```python
from build123d import *

# Parameters (mm, degrees)
SKETCH1_R           = 7.5
SKETCH1_R_2         = 4.5
BOSS_EXTRUDE1_DEPTH = 4
SKETCH3_W           = 1.525
SKETCH3_H           = 4
CUT_EXTRUDE1_DEPTH  = 1.075
CIRPATTERN1_COUNT   = 4
SKETCH6_R           = 0.75
CUT_EXTRUDE3_DEPTH  = 5
CIRPATTERN3_COUNT   = 4


with BuildPart() as part:
    # Sketch1 → Boss-Extrude1 (new body)
    with BuildSketch(Plane(origin=(0, 0, 0), x_dir=(1, 0, 0), z_dir=(0, 1, 0))):
        Circle(SKETCH1_R)
        Circle(SKETCH1_R_2, mode=Mode.SUBTRACT)
    extrude(amount=BOSS_EXTRUDE1_DEPTH)

    # Sketch3 → Cut-Extrude1 (cut, symmetric)
    with BuildSketch(Plane(origin=(0, 0, 0), x_dir=(0, 0, -1), z_dir=(1, 0, 0))):
        with Locations((-6.7375, 2)):
            Rectangle(SKETCH3_W, SKETCH3_H)
    cut_extrude1 = extrude(amount=CUT_EXTRUDE1_DEPTH, both=True, mode=Mode.SUBTRACT)

    # CirPattern1: Cut-Extrude1 ×4 about axis
    cirpattern1_axis = Axis((0, 0, 0), (0, 1, 0))
    for i in range(1, CIRPATTERN1_COUNT):
        add(cut_extrude1.rotate(cirpattern1_axis, i * 360 / CIRPATTERN1_COUNT), mode=Mode.SUBTRACT)

    # Sketch6 → Cut-Extrude3 (cut, through all)
    with BuildSketch(Plane.XZ):
        with Locations((4.242640687, 4.242640687)):
            Circle(SKETCH6_R)
    cut_extrude3 = extrude(amount=-CUT_EXTRUDE3_DEPTH, mode=Mode.SUBTRACT)

    # CirPattern3: Cut-Extrude3 ×4 about axis
    cirpattern3_axis = Axis((0, 0, 0), (0, 1, 0))
    for i in range(1, CIRPATTERN3_COUNT):
        add(cut_extrude3.rotate(cirpattern3_axis, i * 360 / CIRPATTERN3_COUNT), mode=Mode.SUBTRACT)


solid = part.part
```
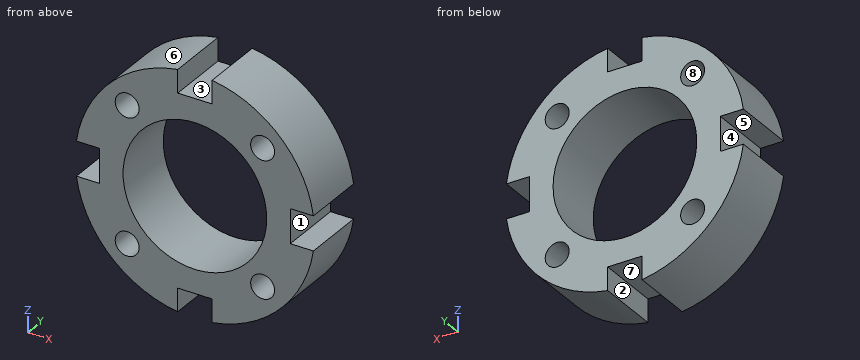
Part model, mm, in its own coordinate system. Face numbers are marked on the shaded views. A direction names the side the tool comes from. Round coordinates to 2 decimals unless told otherwise and drop trailing zeros. Loops run counter-clockwise (first coordinate to the right, second up) from the corner with the lowest first, then second, coordinate; pieces in that order, holes last. Notation, with made-up numbers: (-29.5, 63.5) -> (18.5, 63.5) arc R25 ccw to (18.5, 92.5) -> close; hole circle Ø5 at (76.25, 31.25). An arc over 180 degrees is marked (long way). Use one line per item in the form item = value. Start each with the question number.
Item 1: Two-plate mould, pull along X, no slides. Class the marked faces 5, 6, 7 and 8: released by +X, released by -X, zero draft, split by the parting line, or undercut.
Item 2: Band-saw the part on B-B (x = 0). List the corners of the cut face in (y, z) (3 decimals).
Item 3: Drop flat-ended pins along their axis: pin 1 Ø1.2 at (x, z) = (-4.24, -4.24) entering from -Y; pin 2 Ø1.7 at (y, z) = (2.5, 0.5) entering from +X; pin 3 Ø1.6 at (x, y) = (-6.5, 2.5) entering from +Z; pin 4 Ø0.6 at (x, y) = (0.5, 2) entering from -Z (3 decimals). Give the stop position or say it passes through.
Item 4: Drill centre lines: line 1 along X through (y, z) = (2.45, 4.75); line 2 along X through (y, z) = (0.85, -4). Where is each one in solid material? Low to high.
Item 5: Band-saw the part on C-C (y = 0.75). List the corners of the cut face in (x, z) (3 decimals).
Item 6: Band-saw the part on A-A (z = 0). List the corners of the cut face in (x, y) (3 decimals).
Item 7: Tool access for the marked faces 1, 2, 3 and 4: list every direction of +Z, -Z, +X, -X, +Y, -Y with a clear straight run to the whole face (end or side of a thin tool).
Data:
q1.face_5 = zero draft
q1.face_6 = released by -X
q1.face_7 = undercut
q1.face_8 = undercut
q2.outline = (0, -5.975) -> (4, -5.975) -> (4, -4.5) -> (0, -4.5) -> close; (0, 4.5) -> (4, 4.5) -> (4, 5.975) -> (0, 5.975) -> close
q3.pin_1 = through
q3.pin_2 = 7.42
q3.pin_3 = 4.87
q3.pin_4 = -5.975
q4.line_1 = -5.8 to -4.79, -3.69 to 3.69, 4.79 to 5.8
q4.line_2 = -6.34 to -4.95, -3.53 to -2.06, 2.06 to 3.53, 4.95 to 6.34
q5.outline = (-7.423, -1.075) arc R7.5 ccw to (-1.075, -7.423) -> (-1.075, -5.975) -> (1.075, -5.975) -> (1.075, -7.423) arc R7.5 ccw to (7.423, -1.075) -> (5.975, -1.075) -> (5.975, 1.075) -> (7.423, 1.075) arc R7.5 ccw to (1.075, 7.423) -> (1.075, 5.975) -> (-1.075, 5.975) -> (-1.075, 7.423) arc R7.5 ccw to (-7.423, 1.075) -> (-5.975, 1.075) -> (-5.975, -1.075) -> close; hole circle Ø1.5 at (-4.243, -4.243); hole circle Ø1.5 at (-4.243, 4.243); hole circle Ø9 at (0, 0); hole circle Ø1.5 at (4.243, -4.243); hole circle Ø1.5 at (4.243, 4.243)
q6.outline = (-5.975, 0) -> (-4.5, 0) -> (-4.5, 4) -> (-5.975, 4) -> close; (4.5, 0) -> (5.975, 0) -> (5.975, 4) -> (4.5, 4) -> close
q7.face_1 = +X, +Y, -Y
q7.face_2 = -Z, +Y, -Y
q7.face_3 = +Z, +Y, -Y
q7.face_4 = -X, +Y, -Y
